Read the model definition and answer for the solid it produces. Units are mm, in the model's axes. A direction names the side the tool comes from. Coordinates: 2 decimals unless noted, no trailing zeros. Loops run counter-clockwise (first coordinate to the right, second up) from the corner with the lowest first, then second, coordinate; pieces in that order, holes last. Notation, with made-up numbers: (35, -11.5) -> (74, -11.5) arc R23 cw to (74, 10.5) -> close; hole circle Ø4 at (-5, 54). An arc over 180 degrees is marked (long way). Answer as a JSON object with one key per item and string values. Group by question number.
1) Section B-B, the plane x = -33 is taken. Give the vertices of the cut face in (y, z).
2) Section A-A, the plane y = -60.5 is taken. Give the vertices of the cut face in (x, z).
3) Determine the mould class of faces 1 (the face through (14, 12.813, 1)), 2 (the face through (8.702, -181.436, -4.173)), 3 (the face through (36.281, -84, 0)) for opening direction X: released by +X, released by -X, zero draft, split by the parting line, or undercut.
4) Flat-ended cylindrical pins translate along their axes: P1, Ø1.6, axis at y = 14, z = 0.5, coming from the -X side; P2, Ø1, axis at x = -29.5, z = 0.5, coming from the +Y side; P3, Ø1.5, axis at x = 22, z = -2, coming from the +Y side; P4, Ø3, axis at y = -52.5, z = -5.5, coming from the +X side. Find the tip coordinate at first contact, or state that the pin passes through.
5) Which of the six approach directions +Z, -Z, +X, -X, +Y, -Y give full straight-line access (tool end or side, diameter ignored) to faces 4 (the face through (-49, 12.813, 1)), 5 (the face through (-54.498, -181.436, -4.173)), 6 (the face through (7.181, -180, -2))?
6) Consider probe 1 along X at (y, z) = (-8.5, -1.75); probe 2 along X at (y, z) = (-120, 0.5); probe 3 along Y at (x, z) = (-1, 2.25). Determine where each line is inside the solid, lowest interval first. Write a range as [from, to].
from build123d import *

# Parameters (mm, degrees)
F0_W         = 106
F0_H         = 188.5
F0_W_2       = 90
F0_H_2       = 161.75
F0_H_3       = 7.5
F1_DEPTH     = 3
F2_W         = 3
F2_H         = 7
F3_DEPTH     = 7.75
F4_R         = 3.49999
F5_R         = 1.75
F6_DEPTH     = 86.101
F7_W         = 20
F7_H         = 3
F8_DEPTH     = 10
F9_R         = 3
F10_DEPTH    = 3.001
F11_W        = 2
F11_H        = 196
F12_DEPTH    = 3
F13_R        = 1
F14_R        = 1.75
F15_DEPTH    = 25
F16_T1_DEPTH = 15.5
F16_T4_ANGLE = 90
F16_T6_ANGLE = 90
F18_DEPTH    = 3.0010001
F19_SIZE     = 2


# Not quite as in the source:
# - a fillet or chamfer that OpenCascade refuses, or shapes differently, is made with other operations: its cross-section is extruded or revolved along the edge and cut away or added
# - a fillet or chamfer is up to 0.001 mm smaller than in the source, because OpenCascade refuses the exact size


with BuildPart() as f1:
    # F0 (on Top) → F1 (new body)
    with BuildSketch(Plane.XY):
        with Locations((-16.7186730212, -81.4374315739)):
            Rectangle(F0_W, F0_H)
        with Locations((-16.7186730212, -84.0624315739)):
            Rectangle(F0_W_2, F0_H_2, mode=Mode.SUBTRACT)
        with Locations((-16.7186730212, -179.4374315739)):
            Rectangle(F0_W, F0_H_3)
    extrude(amount=F1_DEPTH)

    # F2 (on face) → F3 (join)
    with BuildSketch(Plane(origin=(0, 0, 0), x_dir=(1, 0, 0), z_dir=(0, 0, -1))):
        with Locations((-48.3186730212, 179.6874315739)):
            Rectangle(F2_W, F2_H)
        with Locations((14.8813269788, 179.6874315739)):
            Rectangle(F2_W, F2_H)
        with Locations((-54.5186730212, 179.6874315739)):
            Rectangle(F2_W, F2_H)
        with Locations((21.0813269788, 179.6874315739)):
            Rectangle(F2_W, F2_H)
        with Locations((-42.1186730212, 179.6874315739)):
            Rectangle(F2_W, F2_H)
        with Locations((8.6813269788, 179.6874315739)):
            Rectangle(F2_W, F2_H)
    extrude(amount=F3_DEPTH)

    # F4 (radius 3.5 in the source; OpenCascade refuses exactly that, so slightly less here)
    f4_edges = [f1.edges().sort_by_distance(p)[0] for p in [
        (-48.318673, -183.187432, -7.75),
        (-48.318673, -176.187432, -7.75),
        (14.881327, -183.187432, -7.75),
        (14.881327, -176.187432, -7.75),
        (-54.518673, -176.187432, -7.75),
        (-54.518673, -183.187432, -7.75),
        (-42.118673, -183.187432, -7.75),
        (-42.118673, -176.187432, -7.75),
        (21.081327, -176.187432, -7.75),
        (8.681327, -176.187432, -7.75),
        (8.681327, -183.187432, -7.75),
        (21.081327, -183.187432, -7.75),
    ]]
    fillet(f4_edges, radius=F4_R)

    # F5 (on face) → F6 (cut, through all)
    with BuildSketch(Plane.YZ.offset(16.3813269788)):
        with Locations((-179.6874315739, -4.25)):
            Circle(F5_R)
    extrude(amount=-F6_DEPTH, mode=Mode.SUBTRACT)

    # F7 (on face) → F8 (join)
    with BuildSketch(Plane(origin=(0, 12.8125684261, 0), x_dir=(-1, 0, 0), z_dir=(0, 1, 0))):
        with Locations((16.7186730212, 1.5)):
            Rectangle(F7_W, F7_H)
    extrude(amount=F8_DEPTH)

    # F9 (on face) → F10 (cut, through all)
    with BuildSketch(Plane(origin=(0, 0, 0), x_dir=(1, 0, 0), z_dir=(0, 0, -1))):
        with Locations((-16.7186730212, -15.8125684261)):
            Circle(F9_R)
    extrude(amount=-F10_DEPTH, mode=Mode.SUBTRACT)

    # F11 (on face) → F12 (join)
    with BuildSketch(Plane(origin=(0, 0, 0), x_dir=(1, 0, 0), z_dir=(0, 0, -1))):
        with Locations((35.2813269788, 85.1874315739)):
            Rectangle(F11_W, F11_H)
        with Locations((-68.7186730212, 85.1874315739)):
            Rectangle(F11_W, F11_H)
    extrude(amount=F12_DEPTH)

    # F13
    f13_edges = [f1.edges().sort_by_distance(p)[0] for p in [
        (14.781327, 12.812568, 3),
        (36.281327, -85.187432, 3),
        (-6.718673, 17.812568, 3),
        (-16.718673, -183.187432, 3),
        (-16.718673, 22.812568, 3),
        (-69.718673, -85.187432, 3),
        (-26.718673, 17.812568, 3),
        (-48.218673, 12.812568, 3),
        (-16.718673, -3.187432, 3),
        (-61.718673, -84.062432, 3),
        (28.281327, -84.062432, 3),
        (-16.718673, -164.937432, 3),
        (-19.718673, 15.812568, 3),
    ]]
    fillet(f13_edges, radius=F13_R)

    # F14 (on face) → F15 (cut)
    with BuildSketch(Plane.YZ.offset(22.5813269788)):
        with Locations((-179.6874315739, -4.25)):
            Circle(F14_R)
    extrude(amount=-F15_DEPTH, mode=Mode.SUBTRACT)

    # F16: fillet of radius 5 on 2 edges, made by hand

    # F16_s2 → F16_t1 (cut)
    with BuildSketch(Plane.XY.offset(-12.5)):
        with BuildLine():
            ThreePointArc((-11.7186730212, 22.8125684261), (-8.1831391152, 21.3481023321), (-6.7186730212, 17.8125684261))
            Line((-6.7186730212, 17.8125684261), (-6.7186730212, 22.8125684261))
            Line((-6.7186730212, 22.8125684261), (-11.7186730212, 22.8125684261))
        make_face()
        with BuildLine():
            ThreePointArc((-26.7186730212, 17.8125684261), (-25.2542069271, 21.3481023321), (-21.7186730212, 22.8125684261))
            Line((-21.7186730212, 22.8125684261), (-26.7186730212, 22.8125684261))
            Line((-26.7186730212, 22.8125684261), (-26.7186730212, 17.8125684261))
        make_face()
    extrude(amount=F16_T1_DEPTH, mode=Mode.SUBTRACT)

    # F16_s3 → F16_t4 (revolve, cut)
    with BuildSketch(Plane.YZ.offset(-21.7186730212)):
        with BuildLine():
            ThreePointArc((21.8125684261, 3), (22.5196752073, 2.7071067812), (22.8125684261, 2))
            Line((22.8125684261, 2), (22.8125684261, 3))
            Line((22.8125684261, 3), (21.8125684261, 3))
        make_face()
    revolve(axis=Axis((-21.7186730212, 17.8125684261, 3), (0, 0, 1)), revolution_arc=F16_T4_ANGLE, mode=Mode.SUBTRACT)

    # F16_s5 → F16_t6 (revolve, cut)
    with BuildSketch(Plane.XZ.offset(-17.8125684261)):
        with BuildLine():
            ThreePointArc((-7.7186730212, 3), (-7.01156624, 2.7071067812), (-6.7186730212, 2))
            Line((-6.7186730212, 2), (-6.7186730212, 3))
            Line((-6.7186730212, 3), (-7.7186730212, 3))
        make_face()
    revolve(axis=Axis((-11.7186730212, 17.8125684261, 3), (0, 0, 1)), revolution_arc=F16_T6_ANGLE, mode=Mode.SUBTRACT)

    # F17 (on face) → F18 (cut, through all)
    with BuildSketch(Plane(origin=(0, 0, 0), x_dir=(1, 0, 0), z_dir=(0, 0, -1))):
        with BuildLine():
            Line((9.8913780288, -0.8125684261), (-43.3287240711, -0.8125684261))
            ThreePointArc((-43.3287240711, -0.8125684261), (-44.3115663992, -1.2196750481), (-44.7186730212, -2.2025173761))
            Line((-44.7186730212, -2.2025173761), (-44.7186730212, -5.4226194761))
            ThreePointArc((-44.7186730212, -5.4226194761), (-44.3115663992, -6.4054618042), (-43.3287240711, -6.8125684261))
            Line((-43.3287240711, -6.8125684261), (9.8913780288, -6.8125684261))
            ThreePointArc((9.8913780288, -6.8125684261), (10.8742203569, -6.4054618042), (11.2813269788, -5.4226194761))
            Line((11.2813269788, -5.4226194761), (11.2813269788, -2.2025173761))
            ThreePointArc((11.2813269788, -2.2025173761), (10.8742203569, -1.2196750481), (9.8913780288, -0.8125684261))
        make_face()
    extrude(amount=-F18_DEPTH, mode=Mode.SUBTRACT)

    # F19
    f19_edges = [f1.edges().sort_by_distance(p)[0] for p in [
        (-16.718673, 6.812568, 3),
    ]]
    chamfer(f19_edges, length=F19_SIZE)


solid = f1.part
Determined:
{
 "1": {"outline": "(-183.19, 0) -> (-164.94, 0) -> (-164.94, 2) arc R1 ccw to (-165.94, 3) -> (-182.19, 3) arc R1 ccw to (-183.19, 2) -> close; (-3.19, 0) -> (0.81, 0) -> (0.81, 1) -> (-1.19, 3) -> (-2.19, 3) arc R1 ccw to (-3.19, 2) -> close; (6.81, 0) -> (12.81, 0) -> (12.81, 2) arc R1 ccw to (11.81, 3) -> (8.81, 3) -> (6.81, 1) -> close"},
 "2": {"outline": "(-69.72, -3) -> (-67.72, -3) -> (-67.72, 0) -> (-61.72, 0) -> (-61.72, 2) arc R1 ccw to (-62.72, 3) -> (-68.72, 3) arc R1 ccw to (-69.72, 2) -> close; (28.28, 0) -> (34.28, 0) -> (34.28, -3) -> (36.28, -3) -> (36.28, 2) arc R1 ccw to (35.28, 3) -> (29.28, 3) arc R1 ccw to (28.28, 2) -> close"},
 "3": {"face 1": "zero draft", "face 2": "undercut", "face 3": "released by +X"},
 "4": {"P1": "x = -26.72", "P2": "y = 12.81", "P3": "y = -176.19", "P4": "through"},
 "5": {"face 4": "+Z, -Z, -X, +Y", "face 5": "none", "face 6": "-Z, +Y, -Y"},
 "6": {"probe 1": "[-69.72, -67.72], [34.28, 36.28]", "probe 2": "[-69.72, -61.72], [28.28, 36.28]", "probe 3": "[-183.16, -164.97], [-3.16, -0.44], [8.06, 12.78]"}
}
